Verification items for the finished model (mm, model axes). Round coordinates to 2 decimals unless told otherwise and drop trailing zeros. Write each loop counter-clockwise with the first axis right and the second up, starting at its lowest first coordinate (ties: lowest second). Pieces come first, ordered by that corner, then holes. Notation, with made-up numbers: (61.5, 69.25) -> (67.5, 69.25) arc R33 ccw to (67.5, 97.25) -> close; hole circle Ø10 at (-23.5, 45.25). An arc over 180 degrees is marked (long way). Use CSV: the item, a comma, the result in double quotes.
```python
from build123d import *

# Parameters (mm, degrees)
F0_W     = 50.8
F0_H     = 38.1
F1_DEPTH = 12.7
F2_R     = 5.08
F3_R     = 6.35
F4_DEPTH = 12.701


with BuildPart() as f1:
    # F0 (on Top) → F1 (new body)
    with BuildSketch(Plane.XY):
        with Locations((0.445614, -19.05)):
            Rectangle(F0_W, F0_H)
    extrude(amount=F1_DEPTH)

    # F2
    f2_edges = [f1.edges().sort_by_distance(p)[0] for p in [
        (-24.954386, -38.1, 6.35),
        (25.845614, -38.1, 6.35),
    ]]
    fillet(f2_edges, radius=F2_R)

    # F3 (on Top) → F4 (cut, through all)
    with BuildSketch(Plane.XY):
        with Locations((0, -25.40782)):
            Circle(F3_R)
    extrude(amount=F4_DEPTH, mode=Mode.SUBTRACT)


solid = f1.part
```
Q1. Mould release check, pull along X, two halves, no side actions. Record for faces 1 (the cylindrical face through (-0.827, -19.112, 6.261)), 2 (the flat face through (0.1, -18.8, 0)), 3 (the flat face through (25.846, -17, 6)): released by +X, released by -X, zero draft, split by the parting line, or undercut.
Filled in:
face 1,"undercut"
face 2,"zero draft"
face 3,"released by +X"
Q2. Section check B-B (y = -28.5). Record the cut outline in (x, z).
Filled in:
outline,"(-24.95, 0) -> (-5.55, 0) -> (-5.55, 12.7) -> (-24.95, 12.7) -> close; (5.55, 0) -> (25.85, 0) -> (25.85, 12.7) -> (5.55, 12.7) -> close"
Q3. Section check C-C (z = 7.25). Record the cut outline in (x, y), plus the area to 3 significant figures.
Filled in:
outline,"(-24.95, -33.02) arc R5.08 ccw to (-19.87, -38.1) -> (20.77, -38.1) arc R5.08 ccw to (25.85, -33.02) -> (25.85, 0) -> (-24.95, 0) -> close; hole circle Ø12.7 at (0, -25.41)"
area,"1,800 mm²"
Q4. Material ranges on L1, parallel to Y at x = 0, z = 3.5; L2, parallel to X at y = -30.5, z = 4.25; L3, parallel to Y at x = -3, z = 8.5, recorded low to high.
Filled in:
L1,"-38.1 to -31.76, -19.06 to 0"
L2,"-24.95 to -3.79, 3.79 to 25.85"
L3,"-38.1 to -31, -19.81 to 0"
Q5. Section check A-A (x = 0). Record the cut outline in (y, z).
Filled in:
outline,"(-38.1, 0) -> (-31.76, 0) -> (-31.76, 12.7) -> (-38.1, 12.7) -> close; (-19.06, 0) -> (0, 0) -> (0, 12.7) -> (-19.06, 12.7) -> close"
